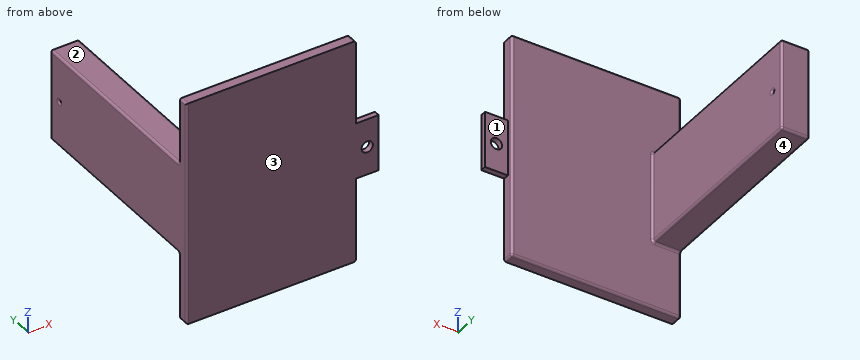
from build123d import *

# Parameters (mm, degrees)
ESQUISSE2_W                  = 150
ESQUISSE2_H                  = 200
BOSS_EXTRU_2_DEPTH           = 10
ESQUISSE3_W                  = 25
ESQUISSE3_H                  = 80.898254602
BOSS_EXTRU_3_DEPTH           = 165
ESQUISSE7_W                  = 50
ESQUISSE7_H                  = 5
BOSS_EXTRU_4_DEPTH           = 95.2
ENL_V_MAT_EXTRU_2_DEPTH      = 95.2
ENL_V_MAT_EXTRU_2_DEPTH_BACK = 95.2
ESQUISSE8_R                  = 5
ESQUISSE9_W                  = 25
ESQUISSE9_H                  = 80.898254602
BOSS_EXTRU_5_DEPTH           = 185.2
ESQUISSE10_R                 = 1.125
ENL_V_MAT_EXTRU_3_DEPTH      = 185.2
CONG_1_R                     = 2


with BuildPart() as part:
    # Esquisse2 → Boss.-Extru.2 (new body)
    with BuildSketch(Plane(origin=(0, 0, 0), x_dir=(1, 0, 0), z_dir=(0, 1, 0))):
        Rectangle(ESQUISSE2_W, ESQUISSE2_H)
    extrude(amount=BOSS_EXTRU_2_DEPTH)

    # Esquisse3 → Boss.-Extru.3 (add)
    with BuildSketch(Plane(origin=(0, 0, 0), x_dir=(1, 0, 0), z_dir=(0, 1, 0))):
        with Locations((-62.5, 0)):
            Rectangle(ESQUISSE3_W, ESQUISSE3_H)
    extrude(amount=BOSS_EXTRU_3_DEPTH)

    # Esquisse7 → Boss.-Extru.4 (add)
    with BuildSketch(Plane(origin=(0, 0, 0), x_dir=(0, 0, -1), z_dir=(1, 0, 0))):
        with Locations((0, 2.5)):
            Rectangle(ESQUISSE7_W, ESQUISSE7_H)
    extrude(amount=BOSS_EXTRU_4_DEPTH)

    # Esquisse8 → Enlèv. mat.-Extru.2 (cut, two sides: drawn at the far end of the back side and taken through both)
    with BuildSketch(Plane(origin=(0, 0, 0), x_dir=(1, 0, 0), z_dir=(0, 1, 0)).offset(-ENL_V_MAT_EXTRU_2_DEPTH_BACK)):
        with Locations(Location((85.1, 0, 0), (0, 0, 90))):
            Circle(ESQUISSE8_R)
    extrude(amount=ENL_V_MAT_EXTRU_2_DEPTH + ENL_V_MAT_EXTRU_2_DEPTH_BACK, mode=Mode.SUBTRACT)

    # Esquisse9 → Boss.-Extru.5 (add)
    with BuildSketch(Plane(origin=(0, 0, 0), x_dir=(1, 0, 0), z_dir=(0, 1, 0))):
        with Locations((-62.5, 0)):
            Rectangle(ESQUISSE9_W, ESQUISSE9_H)
    extrude(amount=BOSS_EXTRU_5_DEPTH)

    # Esquisse10 → Enlèv. mat.-Extru.3 (cut)
    with BuildSketch(Plane(origin=(0, 0, 0), x_dir=(0, 0, -1), z_dir=(1, 0, 0))):
        with Locations((0, 172.95)):
            Circle(ESQUISSE10_R)
    extrude(amount=-ENL_V_MAT_EXTRU_3_DEPTH, mode=Mode.SUBTRACT)

    # Congé1
    cong_1_edges = [part.edges().sort_by_distance(p)[0] for p in [
        (75, 10, 0),
        (-75, 10, 70.224563651),
        (0, 10, -100),
        (-62.5, 10, -40.449127301),
        (-62.5, 10, 40.449127301),
        (-50, 10, 0),
        (-50, 97.6, -40.449127301),
        (-75, 97.6, -40.449127301),
        (-75, 97.6, 40.449127301),
        (-50, 97.6, 40.449127301),
        (-75, 10, -70.224563651),
        (-75, 0, 0),
        (-50, 185.2, 0),
        (-62.5, 185.2, -40.449127301),
        (-75, 185.2, 0),
        (-62.5, 185.2, 40.449127301),
        (-75, 5, -100),
        (75, 5, -100),
        (75, 5, 100),
        (-75, 5, 100),
        (-50, 172.95, 1.125),
        (-75, 172.95, 1.125),
        (0, 10, 100),
    ]]
    fillet(cong_1_edges, radius=CONG_1_R)


solid = part.part
Source: CAD feature listing. Evaluate the final solid. Frame: model axes, mm. Face numbers are marked on the shaded views. A direction names the side the tool comes from. Round coordinates to 2 decimals unless told otherwise and drop trailing zeros. Loops run counter-clockwise (first coordinate to the right, second up) from the corner with the lowest first, then second, coordinate; pieces in that order, holes last. Notation, with made-up numbers: (18, 7) - (77, 7) arc R24 ccw to (77, 41) - close; hole circle Ø5 at (63, 74.5). An arc over 180 degrees is marked (long way). Write item = value, one per line. Start each with the question number.
Item 1: Section query A-A on x = 85.1. Output: boundary loops of the cut face in (y, z).
Item 2: Section query B-B on z = 30. Output: boundary loops of the cut face in (x, y), plus the area to 3 significant figures.
Item 3: Section query C-C on y = 58. Output: boundary loops of the cut face in (x, z).
Item 4: Material intervals for line 1 (X direction, y = 1.6, z = 0); line 2 (Y direction, x = -64.25, z = 0) (3 decimals); line 3 (X direction, y = 174, z = 24.5), sorted ascending.
Item 5: First-contact query: pin 1 Ø10.5 at (x, y) = (-58, 133) entering from -Z; pin 2 Ø4 at (x, y) = (87.5, 3.5) entering from +Z; pin 3 Ø17 at (x, y) = (-66.5, 89) entering from +Z; pin 4 Ø9 at (y, z) = (5.5, -19.5) entering from +X. Flat tips, straight axial feed; report the tip coordinate or a pass-through.
Item 6: Reachability of the marked faces 1, 2, 3 and 4 from +Z, -Z, +X, -X, +Y, -Y: full face, straight path, thin tool, end or side. Return the list, or none.
Item 7: Section query D-D on x = -9. Output: boundary loops of the cut face in (y, z), plus the area to 3 significant figures.
Results list:
q1.outline = (0, -25) - (5, -25) - (5, -5) - (0, -5) - close; (0, 5) - (5, 5) - (5, 25) - (0, 25) - close
q2.outline = (-75, 2) arc R2 ccw to (-73, 0) - (75, 0) - (75, 8) arc R2 ccw to (73, 10) - (-48, 10) arc R2 cw to (-50, 12) - (-50, 183.2) arc R2 ccw to (-52, 185.2) - (-73, 185.2) arc R2 ccw to (-75, 183.2) - close
q2.area = 5,880 mm²
q3.outline = (-75, -38.45) arc R2 ccw to (-73, -40.45) - (-52, -40.45) arc R2 ccw to (-50, -38.45) - (-50, 38.45) arc R2 ccw to (-52, 40.45) - (-73, 40.45) arc R2 ccw to (-75, 38.45) - close
q4.line_1 = -74.96 to 80.1, 90.1 to 95.2
q4.line_2 = 0 to 171.825, 174.075 to 185.2
q4.line_3 = -75 to -50
q5.pin_1 = -40.45
q5.pin_2 = 25
q5.pin_3 = 40.45
q5.pin_4 = 95.2
q6.face_1 = +Z, -Z, +X, +Y
q6.face_2 = +Z, +X, -X, +Y
q6.face_3 = +Z, -Z, +X, -X, -Y
q6.face_4 = -Z, +X, -X, +Y
q7.outline = (0, -100) - (8, -100) arc R2 ccw to (10, -98) - (10, 98) arc R2 ccw to (8, 100) - (0, 100) - close
q7.area = 2,000 mm²
